The drawing under review shows one solid part. Ordinate dimensions are in mm from its lowest x, y, z. Give positions to 0.01 mm unless a question says otherwise; leave off trailing zeros. Write each loop counter-clockwise with the first axis right and the second up, starting at its lowest first coordinate (ties: lowest second). Pieces come first, ordered by that corner, then holes. Notation, with made-up numbers: (-25, 48) - (11, 48) arc R24 cw to (11, 78) - close; hole circle Ø11 at (8.5, 35.25). An arc over 180 degrees is marked (long way). Write each question's results on one line, items separated by ' | '. Start each with the question number.
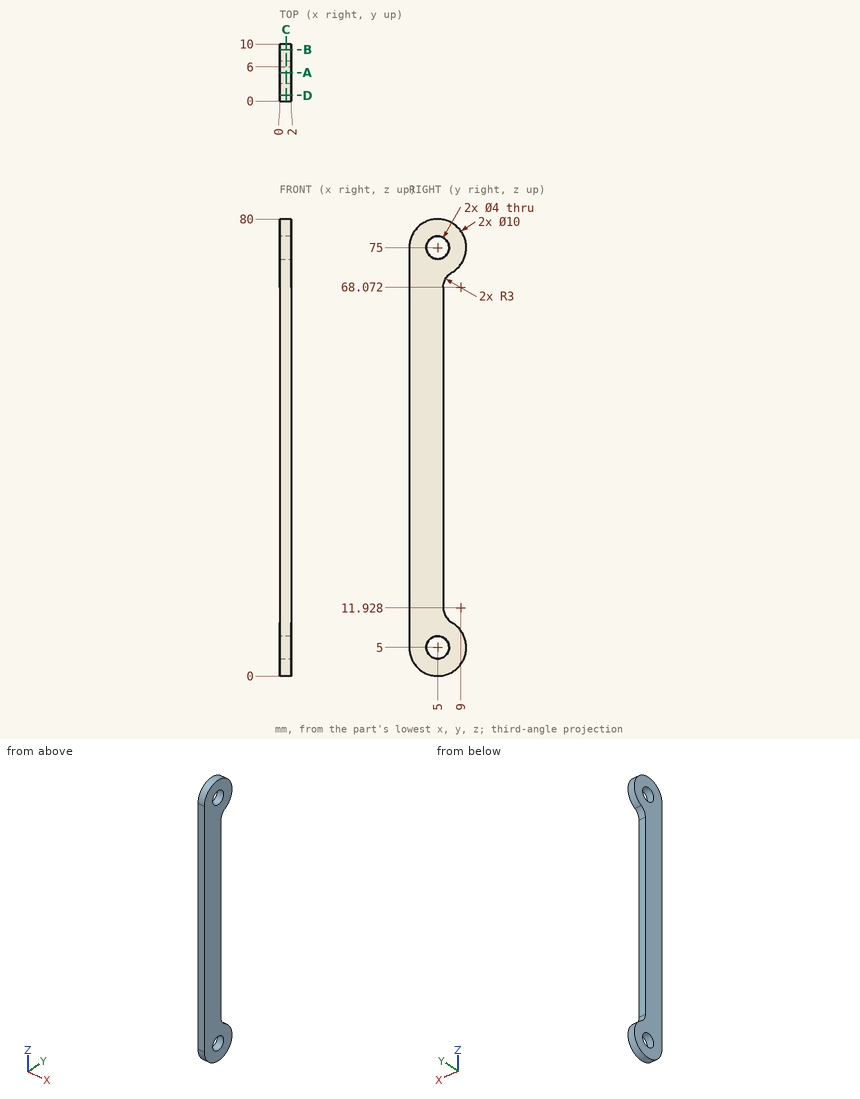
Q1. Add section D-D on y = 1. State the section outline as (x, z) points.
Q2. Add section C-C on x = 1.1. State the section outline as (y, z) points, plus the area to 3 significant figures.
Q3. For line 1 along Z through (x, y) = (0.9, 5); line 2 along Z through (x, y) = (0.8, 6.5); line 3 along Y through (x, z) = (1.45, 5), list the stretches that pass through material, from the lowest coordinate up. Write a range as [from, to].
Q4. Add section B-B on y = 9. State the section outline as (x, z) points, plus the area to 3 significant figures.
Q5. Insertion check: P1, Ø0.6, axis at x = 0.5, z = 45.5, coming from the +Y side. The pin has a flat end and moves straight along its axis. Give the tip position at first contact, or say it passes through.
Q6. Add section A-A on y = 5. State the section outline as (x, z) points, plus the area to 3 significant figures.
Result:
1) outline: (0, 2) - (2, 2) - (2, 78) - (0, 78) - close
2) outline: (0, 5) arc R5 ccw (long way) to (7.5, 9.33) arc R3 cw to (6, 11.93) - (6, 68.07) arc R3 cw to (7.5, 70.67) arc R5 ccw (long way) to (0, 75) - close; hole circle Ø4 at (5, 5); hole circle Ø4 at (5, 75) | area: 504 mm²
3) line 1: z = [0, 3], [7, 73], [77, 80] | line 2: z = [0.23, 3.68], [6.32, 10.27], [69.73, 73.68], [76.32, 79.77] | line 3: y = [0, 3], [7, 10]
4) outline: (0, 2) - (2, 2) - (2, 8) - (0, 8) - close; (0, 72) - (2, 72) - (2, 78) - (0, 78) - close | area: 24.0 mm²
5) P1: stops at y = 6
6) outline: (0, 0) - (2, 0) - (2, 3) - (0, 3) - close; (0, 7) - (2, 7) - (2, 73) - (0, 73) - close; (0, 77) - (2, 77) - (2, 80) - (0, 80) - close | area: 144 mm²
